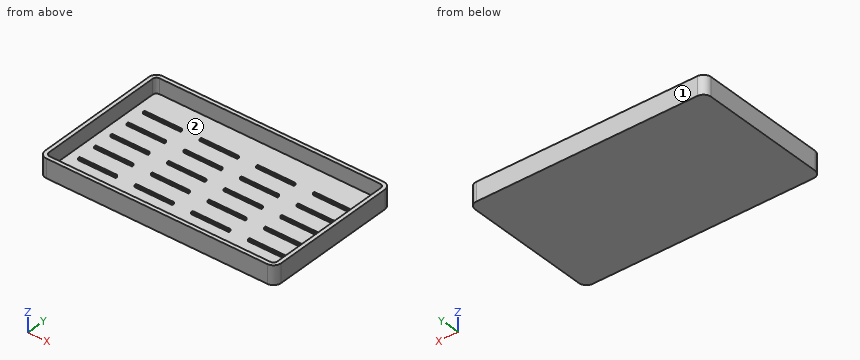
```python
from build123d import *

# Parameters (mm, degrees)
SKETCH1_W           = 125
SKETCH1_H           = 75
BOSS_EXTRUDE1_DEPTH = 10
FILLET1_R           = 4
SHELL1_T            = -2
SKETCH2_W           = 20
SKETCH2_H           = 1
BOSS_EXTRUDE2_DEPTH = 1


with BuildPart() as part:
    # Sketch1 → Boss-Extrude1 (new body)
    with BuildSketch(Plane.XY):
        with Locations((62.5, 37.5)):
            Rectangle(SKETCH1_W, SKETCH1_H)
    extrude(amount=BOSS_EXTRUDE1_DEPTH)

    # Fillet1
    fillet1_edges = [part.edges().sort_by_distance(p)[0] for p in [
        (0, 75, 5),
        (125, 75, 5),
        (125, 0, 5),
        (0, 0, 5),
    ]]
    fillet(fillet1_edges, radius=FILLET1_R)

    # Shell1
    shell1_openings = [part.faces().sort_by_distance(p)[0] for p in [
        (62.5, 37.5, 10),
    ]]
    offset(amount=SHELL1_T, openings=shell1_openings, kind=Kind.INTERSECTION)

    # Sketch2 → Boss-Extrude2 (add)
    with BuildSketch(Plane.XY.offset(2)):
        with Locations((107.5, 58.5)):
            Rectangle(SKETCH2_W, SKETCH2_H)
        with Locations((77.5, 58.5)):
            Rectangle(SKETCH2_W, SKETCH2_H)
        with Locations((77.5, 48)):
            Rectangle(SKETCH2_W, SKETCH2_H)
        with Locations((77.5, 37.5)):
            Rectangle(SKETCH2_W, SKETCH2_H)
        with Locations((77.5, 27)):
            Rectangle(SKETCH2_W, SKETCH2_H)
        with Locations((77.5, 16.5)):
            Rectangle(SKETCH2_W, SKETCH2_H)
        with Locations((107.5, 48)):
            Rectangle(SKETCH2_W, SKETCH2_H)
        with Locations((107.5, 37.5)):
            Rectangle(SKETCH2_W, SKETCH2_H)
        with Locations((107.5, 27)):
            Rectangle(SKETCH2_W, SKETCH2_H)
        with Locations((107.5, 16.5)):
            Rectangle(SKETCH2_W, SKETCH2_H)
        with Locations((47.5, 58.5)):
            Rectangle(SKETCH2_W, SKETCH2_H)
        with Locations((47.5, 48)):
            Rectangle(SKETCH2_W, SKETCH2_H)
        with Locations((47.5, 37.5)):
            Rectangle(SKETCH2_W, SKETCH2_H)
        with Locations((47.5, 27)):
            Rectangle(SKETCH2_W, SKETCH2_H)
        with Locations((47.5, 16.5)):
            Rectangle(SKETCH2_W, SKETCH2_H)
        with Locations((17.5, 58.5)):
            Rectangle(SKETCH2_W, SKETCH2_H)
        with Locations((17.5, 48)):
            Rectangle(SKETCH2_W, SKETCH2_H)
        with Locations((17.5, 37.5)):
            Rectangle(SKETCH2_W, SKETCH2_H)
        with Locations((17.5, 27)):
            Rectangle(SKETCH2_W, SKETCH2_H)
        with Locations((17.5, 16.5)):
            Rectangle(SKETCH2_W, SKETCH2_H)
    extrude(amount=BOSS_EXTRUDE2_DEPTH)


solid = part.part
```
Input: part model. Units: mm. Frame: model coordinates. Face numbers are marked on the shaded views. Round coordinates to 2 decimals unless told otherwise and drop trailing zeros. Write each loop counter-clockwise with the first axis right and the second up, starting at its lowest first coordinate (ties: lowest second). Pieces come first, ordered by that corner, then holes. Notation, with made-up numbers: (-3.75, 28) - (1.25, 28) arc R32 cw to (1.25, 54) - close; hole circle Ø9 at (59, 72.5). An arc over 180 degrees is marked (long way). Write item = value, one per line.
(1) Section query C-C on y = 46. Output: boundary loops of the cut face in (x, z), then the cut area to 3 significant figures.
Geometry check:
outline = (0, 0) - (125, 0) - (125, 10) - (123, 10) - (123, 2) - (2, 2) - (2, 10) - (0, 10) - close
area = 282 mm^2
(2) Section query A-A on z = 4.5. Output: boundary loops of the cut face in (x, y), then the cut area to 3 significant figures.
Geometry check:
outline = (0, 4) arc R4 ccw to (4, 0) - (121, 0) arc R4 ccw to (125, 4) - (125, 71) arc R4 ccw to (121, 75) - (4, 75) arc R4 ccw to (0, 71) - close; hole (2, 4) arc R2 ccw to (4, 2) - (121, 2) arc R2 ccw to (123, 4) - (123, 71) arc R2 ccw to (121, 73) - (4, 73) arc R2 ccw to (2, 71) - close
area = 774 mm^2
(3) Material intervals for probe 1 along X at (y, z) = (35.5, 9.25); probe 2 along Y at (x, z) = (19, 7.25); probe 3 along Z at (x, y) = (77, 9.5), sorted ascending.
Geometry check:
probe_1 = 0 to 2, 123 to 125
probe_2 = 0 to 2, 73 to 75
probe_3 = 0 to 2
(4) Section query D-D on x = 100. Output: boundary loops of the cut face in (y, z), then the cut area to 3 significant figures.
Geometry check:
outline = (0, 0) - (75, 0) - (75, 10) - (73, 10) - (73, 2) - (59, 2) - (59, 3) - (58, 3) - (58, 2) - (48.5, 2) - (48.5, 3) - (47.5, 3) - (47.5, 2) - (38, 2) - (38, 3) - (37, 3) - (37, 2) - (27.5, 2) - (27.5, 3) - (26.5, 3) - (26.5, 2) - (17, 2) - (17, 3) - (16, 3) - (16, 2) - (2, 2) - (2, 10) - (0, 10) - close
area = 187 mm^2
(5) Contact query for a flat-ended pin moving along its axis: pin 1 Ø8 at (x, y) = (63.5, 24.5) entering from +Z. Output: stop coordinate, or through.
Geometry check:
pin_1 = 2
(6) Pull-direction query (X, two-part tool) for the marked faces 1 and 2; classes: +X half, -X half, draft (parallel to the pull), parting line (faces both ways), or undercut.
Geometry check:
face_1 = draft
face_2 = undercut
(7) Section query B-B on x = 59. Output: boundary loops of the cut face in (y, z).
Geometry check:
outline = (0, 0) - (75, 0) - (75, 10) - (73, 10) - (73, 2) - (2, 2) - (2, 10) - (0, 10) - close
